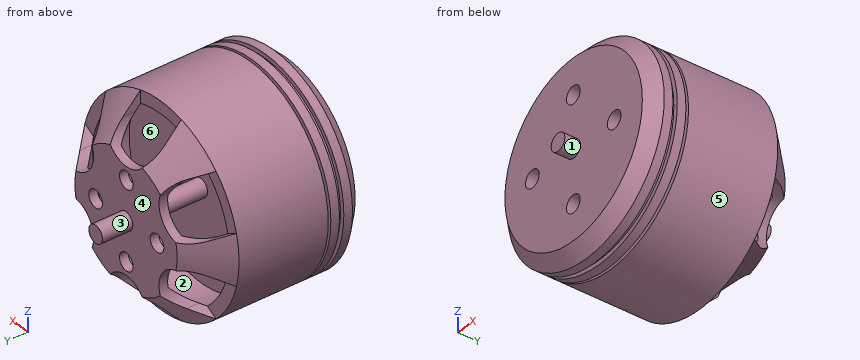
```python
from build123d import *

# Parameters (mm, degrees)
SKETCH2_R          = 1
CUT_EXTRUDE1_DEPTH = 4
SKETCH3_R          = 1
CUT_EXTRUDE2_DEPTH = 3


with BuildPart() as part:
    # Sketch1 → Revolve1 (revolve)
    with BuildSketch(Plane.XY):
        Polygon((0.048979582, -2.362225903), (1.048979582, -2.362225903), (1.048979582, -0.562225903), (10.134766019, -0.562225903), (11.548979582, 0.85198766), (11.548979582, 1.85198766), (11.048979582, 1.85198766), (11.048979582, 2.35198766), (11.548979582, 2.35198766), (11.548979582, 3.35198766), (9.548979582, 3.35198766), (9.548979582, 3.65198766), (11.548979582, 3.65198766), (11.548979582, 13.937774097), (7.548979582, 17.937774097), (1.048979582, 17.937774097), (1.048979582, 21.437774097), (0.048979582, 21.437774097), align=None)
        Polygon((2.048979582, 16.937774097), (7.134766019, 16.937774097), (10.548979582, 13.523560535), (10.548979582, 9.305259573), (1.048979582, 9.305259573), (1.048979582, 15.937774097), (2.048979582, 15.937774097), align=None, mode=Mode.SUBTRACT)
    revolve(axis=Axis((0.048979582, 21.437774097, 0), (0, -1, 0)))

    # Sketch2 → Cut-Extrude1 (cut)
    with BuildSketch(Plane(origin=(0, 17.937774097, 0), x_dir=(1, 0, 0), z_dir=(0, 1, 0))):
        with Locations((0, 4.5)):
            Circle(SKETCH2_R)
        with Locations((4.5, 0)):
            Circle(SKETCH2_R)
        with Locations((0, -4.5)):
            Circle(SKETCH2_R)
        with Locations((-4.5, 0)):
            Circle(SKETCH2_R)
        with BuildLine():
            Line((-3, 9), (-3, 17.185640614))
            Line((-3, 17.185640614), (3, 17.185640614))
            Line((3, 17.185640614), (3, 9))
            ThreePointArc((3, 9), (0, 6), (-3, 9))
        make_face()
        with BuildLine():
            Line((16.383201352, 5.994744096), (9.294228634, 1.901923789))
            ThreePointArc((9.294228634, 1.901923789), (5.196152423, 3), (6.294228634, 7.098076211))
            Line((6.294228634, 7.098076211), (13.383201352, 11.190896518))
            Line((13.383201352, 11.190896518), (16.383201352, 5.994744096))
        make_face()
        with BuildLine():
            Line((13.383201352, -11.190896518), (6.294228634, -7.098076211))
            ThreePointArc((6.294228634, -7.098076211), (5.196152423, -3), (9.294228634, -1.901923789))
            Line((9.294228634, -1.901923789), (16.383201352, -5.994744096))
            Line((16.383201352, -5.994744096), (13.383201352, -11.190896518))
        make_face()
        with BuildLine():
            Line((-3, -17.185640614), (-3, -9))
            ThreePointArc((-3, -9), (0, -6), (3, -9))
            Line((3, -9), (3, -17.185640614))
            Line((3, -17.185640614), (-3, -17.185640614))
        make_face()
        with BuildLine():
            Line((-16.383201352, -5.994744096), (-9.294228634, -1.901923789))
            ThreePointArc((-9.294228634, -1.901923789), (-5.196152423, -3), (-6.294228634, -7.098076211))
            Line((-6.294228634, -7.098076211), (-13.383201352, -11.190896518))
            Line((-13.383201352, -11.190896518), (-16.383201352, -5.994744096))
        make_face()
        with BuildLine():
            Line((-13.383201352, 11.190896518), (-6.294228634, 7.098076211))
            ThreePointArc((-6.294228634, 7.098076211), (-5.196152423, 3), (-9.294228634, 1.901923789))
            Line((-9.294228634, 1.901923789), (-16.383201352, 5.994744096))
            Line((-16.383201352, 5.994744096), (-13.383201352, 11.190896518))
        make_face()
    extrude(amount=-CUT_EXTRUDE1_DEPTH, mode=Mode.SUBTRACT)

    # Sketch3 → Cut-Extrude2 (cut)
    with BuildSketch(Plane.XZ.offset(0.562225903)):
        with Locations((0, 6)):
            Circle(SKETCH3_R)
        with Locations((6, 0)):
            Circle(SKETCH3_R)
        with Locations((0, -6)):
            Circle(SKETCH3_R)
        with Locations((-6, 0)):
            Circle(SKETCH3_R)
    extrude(amount=-CUT_EXTRUDE2_DEPTH, mode=Mode.SUBTRACT)


solid = part.part
```
Geometry: final body of the model. Coordinates: model frame, mm. Face numbers are marked on the shaded views. A direction names the side the tool comes from. Round coordinates to 2 decimals unless told otherwise and drop trailing zeros. Order: outer loops, then holes, each group sorted by start corner. A loop starts at its lowest first (then second) coordinate and runs counter-clockwise, first axis right, second up. Notation, with made-up numbers: M 48.5,21.25 L 99.5,21.25 A21 ccw 99.5,48.25 Z; hole C 49,15 d5. An arc over 180 degrees is marked long. One line per item, written item: value.
(1) Cut plane B-B (y = 4.25). Return the cut outline in (x, z).
Result sheet:
outline: C 0.05,0 d23
(2) Reachability of the marked faces 1, 2 and 3 from +Z, -Z, +X, -X, +Y, -Y: full face, straight path, thin tool, end or side. Return the list, or none.
Result sheet:
face 1: -Y
face 2: none
face 3: +Y
(3) Line query: probe 1 along Z at (x, y) = (0, 17.4); probe 2 along Y at (x, z) = (-5, 1.25); probe 3 along Y at (x, z) = (3.5, 9.5). Output: solid intervals per line, ascending. Write a range as [from, to].
Result sheet:
probe 1: [-6, -5.5], [-3.5, 3.5], [5.5, 6]
probe 2: [-0.56, 9.31], [16.94, 17.94]
probe 3: [-0.54, 3.35], [3.65, 9.31], [13.92, 15.33]
(4) Pin query (flat end, axial travel): P1, Ø0.6, axis at x = -6, z = 0, coming from the -Y side; P2, Ø7, axis at x = 1, z = 1, coming from the -Y side; P3, Ø1.6, axis at x = -4.5, z = 0, coming from the -Y side; P4, Ø2, axis at x = -0.5, z = -10.5, coming from the +Y side. Return the tip coordinate at first contact, or that it passes through.
Result sheet:
P1: y = 2.44
P2: y = -2.36
P3: y = -0.56
P4: y = 13.94
(5) Pull-direction query (X, two-part tool) for the marked faces 4, 5 and 6; classes: pulls with the +X half, pulls with the -X half, needs draft (parallel to the pull), parting line crosses it, or undercut.
Result sheet:
face 4: needs draft
face 5: parting line crosses it
face 6: undercut
(6) Cut plane A-A (x = 0). Give the number of separate pieces and of enclosed holes in the cut face, and give its area (3 significant figures).
Result sheet:
separate pieces: 3
enclosed holes: 0
area: 257 mm2
